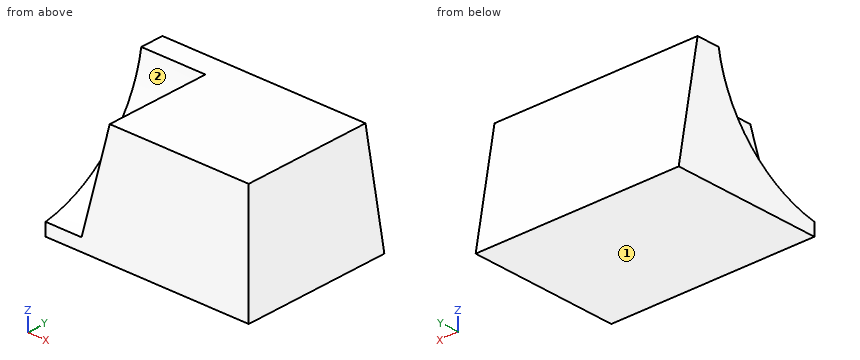
```python
from build123d import *

# Parameters (mm, degrees)
F0_W     = 190
F0_H     = 120
F1_DEPTH = 110
F3_DEPTH = 190
F7_REACH = 199.0477340594


with BuildPart() as f1:
    # F0 (on Top) → F1 (new body)
    with BuildSketch(Plane.XY):
        Rectangle(F0_W, F0_H)
    extrude(amount=-F1_DEPTH)

    # F2 (on face) → F3 (join, through all)
    with BuildSketch(Plane.YZ.offset(95)):
        Polygon((79.3959678779, -110), (60, 0), (60, -110), align=None)
    extrude(amount=-F3_DEPTH)

    f7_end = Plane(origin=(-32.6554445662, 0, 8.75), x_dir=(0.2588190451, 0, 0.9659258263), z_dir=(0.9659258263, 0, -0.2588190451))
    # F4 (on face) → F7 (cut, up to a plane its end follows)
    with BuildSketch(Plane(origin=(-95, 0, 0), x_dir=(0, -1, 0), z_dir=(-1, 0, 0))):
        with BuildLine():
            Line((60, -98.321595662), (60, 0))
            Line((60, 0), (-38.321595662, 0))
            ThreePointArc((-38.321595662, 0), (-4.8528137424, -64.8528137424), (60, -98.321595662))
        make_face()
    f7_long = extrude(amount=-F7_REACH, mode=Mode.PRIVATE)
    add(split(f7_long, bisect_by=f7_end, keep=Keep.BOTTOM, mode=Mode.PRIVATE), mode=Mode.SUBTRACT)


solid = f1.part
```
Source: CAD feature listing. Evaluate the final solid. Frame: model axes, mm. Face numbers are marked on the shaded views. A direction names the side the tool comes from. Give positions to 0.01 mm unless a question says otherwise; leave off trailing zeros. Loops run counter-clockwise (first coordinate to the right, second up) from the corner with the lowest first, then second, coordinate; pieces in that order, holes last. Notation, with made-up numbers: (6, -36.5) -> (65, -36.5) arc R18 cw to (65, -28.5) -> close; hole circle Ø9 at (9, -6.5). An arc over 180 degrees is marked (long way). Use a Markdown table: item, result. Add a question column.
(1) Section query B-B (y = -9). Output: boundary loops of the cut face in (x, z), then the cut area to 3 significant figures.
(2) Ray query, line 1 (Y direction, x = -41, z = -72); line 2 (Z direction, x = -68.5, y = 20); line 3 (Y direction, x = -33.5, z = -39). Return the intervals inside material, ascending.
(3) Access query for the marked faces 1 and 2. Directions: +Z, -Z, +X, -X, +Y, -Y. A direction counts if a zero-diameter tool reaches every point of the face in a straight line with its end or side. Return the directions, or none.
(4) Section query C-C (z = -15.5). Output: boundary loops of the cut face in (x, y), then the cut area to 3 significant figures.
(5) First-contact query: pin 1 Ø1.5 at (x, z) = (-7.5, -95.5) entering from +Y; pin 2 Ø5 at (x, y) = (-67, 7) entering from +Z; pin 3 Ø6 at (y, z) = (-35.5, -17.5) entering from -X. Flat tips, straight axial feed; report the tip coordinate or a pass-through.
(6) Section query A-A (x = -73.5). Output: boundary loops of the cut face in (y, z), then the cut area to 3 significant figures.
(7) Section query D-D (x = -24). Output: boundary loops of the cut face in (y, z).
Checked values:
| question | item | result |
|---|---|---|
| 1 | outline | (-95, -110) -> (95, -110) -> (95, 0) -> (-35, 0) -> (-55.56, -76.74) -> (-95, -76.74) -> close |
| 1 | area | 17,100 mm^2 |
| 2 | line 1 | -60 to 72.7 |
| 2 | line 2 | -110 to -46.33 |
| 2 | line 3 | -60 to 66.88 |
| 3 | face 1 | -Z, +X, -X, +Y, -Y |
| 3 | face 2 | +Z, -X, -Y |
| 4 | outline | (-95, 34.63) -> (-39.15, 34.63) -> (-39.15, -60) -> (95, -60) -> (95, 62.73) -> (-95, 62.73) -> close |
| 4 | area | 18,000 mm^2 |
| 5 | pin 1 | y = 76.97 |
| 5 | pin 2 | z = -59.94 |
| 5 | pin 3 | x = -40.49 |
| 6 | outline | (-60, -110) -> (79.4, -110) -> (60, 0) -> (38.32, 0) arc R120 cw to (-60, -98.32) -> close |
| 6 | area | 7,330 mm^2 |
| 7 | outline | (-60, -110) -> (79.4, -110) -> (60, 0) -> (-60, 0) -> close |
